Verification items for the finished model (mm, model axes). Give positions to 0.01 mm unless a question says otherwise; leave off trailing zeros. Order: outer loops, then holes, each group sorted by start corner. A loop starts at its lowest first (then second) coordinate and runs counter-clockwise, first axis right, second up. Notation, with made-up numbers: (-17, 49) - (-12, 49) arc R13 ccw to (-12, 73) - close; hole circle Ø2 at (70.5, 25.5). An arc over 180 degrees is marked (long way). Answer as a JSON object with one key per item and string values. Group by question number.
(1) Section check A-A (y = -33.95). Record the boundary of the cut face in (x, z).
(2) Thickness scan on line 1 (X direction, y = -33.95, z = 0.55); line 2 (X direction, y = -26, z = 1.2); line 3 (Y direction, x = 2, z = -0.75). Record the ranges inside material, lowest first.
(3) Section check B-B (x = 0). Record the boundary of the cut face in (y, z).
(4) Mould release check, pull along Y, two halves, no side actions. Record for faces 1 (the face through (4.116, -33.256, -0.021)), 2 (the face through (-15, 0, 0)), 3 (the face through (0, -35, 0)): +Y half, -Y half, draft (parallel to the pull), parting line (faces both ways), or undercut.
```python
from build123d import *

# Parameters (mm, degrees)
MAINBODY_EXTRUDE_START            = -1.5
PROJECTIONXY_SKETCH_W             = 30
PROJECTIONXY_SKETCH_H             = 70
MAINBODY_EXTRUDE_DEPTH            = 3
BORE_CUT_DEPTH                    = 39.108398025
BORE_CUT_DEPTH_BACK               = 39.108398025
BORE_SKETCH_R                     = 2.55
POSTCLEARANCEHOLES_CUT_DEPTH      = 39.108398025
POSTCLEARANCEHOLES_CUT_DEPTH_BACK = 39.108398025
POSTCLEARANCEHOLES_SKETCH_R       = 0.7


with BuildPart() as part:
    # projectionXy_sketch → mainBody_extrude (new body)
    with BuildSketch(Plane.XY.offset(MAINBODY_EXTRUDE_START)):
        Rectangle(PROJECTIONXY_SKETCH_W, PROJECTIONXY_SKETCH_H)
    extrude(amount=MAINBODY_EXTRUDE_DEPTH)

    # bore_sketch → bore_cut (cut, two sides: drawn at the far end of the back side and taken through both)
    with BuildSketch(Plane.XY.offset(-BORE_CUT_DEPTH_BACK)):
        with Locations((0, -29.742714652)):
            Circle(BORE_SKETCH_R)
    extrude(amount=BORE_CUT_DEPTH + BORE_CUT_DEPTH_BACK, mode=Mode.SUBTRACT)

    # postClearanceHoles_sketch → postClearanceHoles_cut (cut, two sides: drawn at the far end of the back side and taken through both)
    with BuildSketch(Plane.XY.offset(-POSTCLEARANCEHOLES_CUT_DEPTH_BACK)):
        with Locations((4.207285348, -25.535429304)):
            Circle(POSTCLEARANCEHOLES_SKETCH_R)
        with Locations((-4.207285348, -25.535429304)):
            Circle(POSTCLEARANCEHOLES_SKETCH_R)
        with Locations((-4.207285348, -33.95)):
            Circle(POSTCLEARANCEHOLES_SKETCH_R)
        with Locations((4.207285348, -33.95)):
            Circle(POSTCLEARANCEHOLES_SKETCH_R)
    extrude(amount=POSTCLEARANCEHOLES_CUT_DEPTH + POSTCLEARANCEHOLES_CUT_DEPTH_BACK, mode=Mode.SUBTRACT)


solid = part.part
```
Solutions:
{
 "1": {"outline": "(-15, -1.5) - (-4.91, -1.5) - (-4.91, 1.5) - (-15, 1.5) - close; (-3.51, -1.5) - (3.51, -1.5) - (3.51, 1.5) - (-3.51, 1.5) - close; (4.91, -1.5) - (15, -1.5) - (15, 1.5) - (4.91, 1.5) - close"},
 "2": {"line 1": "x = -15 to -4.91, -3.51 to 3.51, 4.91 to 15", "line 2": "x = -15 to -4.73, -3.68 to 3.68, 4.73 to 15", "line 3": "y = -35 to -31.32, -28.16 to 35"},
 "3": {"outline": "(-35, -1.5) - (-32.29, -1.5) - (-32.29, 1.5) - (-35, 1.5) - close; (-27.19, -1.5) - (35, -1.5) - (35, 1.5) - (-27.19, 1.5) - close"},
 "4": {"face 1": "undercut", "face 2": "draft", "face 3": "-Y half"}
}
